from build123d import *

# Parameters (mm, degrees)
MODEL_R                 = 8.05
MODEL_W                 = 5
MODEL_H                 = 5
SALIENTE_EXTRUIR1_DEPTH = 3
CROQUIS3_W              = 20
CROQUIS3_H              = 3
SALIENTE_EXTRUIR2_DEPTH = 8
CROQUIS4_R              = 1.5
CORTAR_EXTRUIR1_DEPTH   = 3
CROQUIS5_R              = 2.25
CORTAR_EXTRUIR2_DEPTH   = 1
REDONDEO1_R             = 2
CROQUIS6_R              = 12
CORTAR_EXTRUIR3_DEPTH   = 1


with BuildPart() as part:
    # Model → Saliente-Extruir1 (new body)
    with BuildSketch(Plane.XY):
        with BuildLine():
            Line((50.698959582, -56.020997464), (70.698959582, -56.020997464))
            Line((70.698959582, -56.020997464), (70.698959582, -55.020997464))
            ThreePointArc((70.698959582, -55.020997464), (71.28474602, -53.606783901), (72.698959582, -53.020997464))
            Line((72.698959582, -53.020997464), (88.870799912, -53.020997464))
            ThreePointArc((88.870799912, -53.020997464), (90.285013474, -52.435211026), (90.870799912, -51.020997464))
            Line((90.870799912, -51.020997464), (90.870799912, 1.979002536))
            ThreePointArc((90.870799912, 1.979002536), (90.150187884, 3.212884764), (88.940527152, 3.973455574))
            ThreePointArc((88.940527152, 3.973455574), (82.556801864, 7.967186508), (80.592387516, 15.236499516))
            ThreePointArc((80.592387516, 15.236499516), (73.016137183, 12.831206377), (66.424253692, 8.389126209))
            ThreePointArc((66.424253692, 8.389126209), (62.464845981, 11.66270114), (60.387431279, 16.361376528))
            ThreePointArc((60.387431279, 16.361376528), (55.039384462, 14.426569266), (50.461877073, 11.051438157))
            ThreePointArc((50.461877073, 11.051438157), (49.41482724, 13.546636971), (50.438823204, 16.051385009))
            ThreePointArc((50.438823204, 16.051385009), (43.800023098, 13.634815248), (38.471226177, 8.99613013))
            ThreePointArc((38.471226177, 8.99613013), (37.976525569, 11.673196605), (38.618250464, 14.318872844))
            ThreePointArc((38.618250464, 14.318872844), (33.077419178, 10.94136051), (30.527119253, 4.974420659))
            Line((30.527119253, 4.974420659), (30.527119253, -51.020997464))
            ThreePointArc((30.527119253, -51.020997464), (31.112905691, -52.435211026), (32.527119253, -53.020997464))
            Line((32.527119253, -53.020997464), (48.698959582, -53.020997464))
            ThreePointArc((48.698959582, -53.020997464), (50.113173145, -53.606783901), (50.698959582, -55.020997464))
            Line((50.698959582, -55.020997464), (50.698959582, -56.020997464))
        make_face()
        with Locations((47.698959583, -8.020997464)):
            Circle(MODEL_R, mode=Mode.SUBTRACT)
        with Locations((73.698959582, -8.020997464)):
            Circle(MODEL_R, mode=Mode.SUBTRACT)
        Polygon((53.283896073, -43.364264203), (57.614023092, -45.864264203), (60.114023092, -41.534137185), (55.783896073, -39.034137185), align=None, mode=Mode.SUBTRACT)
        Polygon((63.783896073, -45.864264204), (68.114023092, -43.364264204), (65.614023092, -39.034137185), (61.283896073, -41.534137185), align=None, mode=Mode.SUBTRACT)
        with Locations((68.698959582, -35.520997464)):
            Rectangle(MODEL_W, MODEL_H, mode=Mode.SUBTRACT)
        Polygon((68.114023092, -27.677730724), (63.783896073, -25.177730724), (61.283896073, -29.507857743), (65.614023092, -32.007857743), align=None, mode=Mode.SUBTRACT)
        Polygon((57.614023092, -25.177730724), (53.283896073, -27.677730724), (55.783896073, -32.007857743), (60.114023092, -29.507857743), align=None, mode=Mode.SUBTRACT)
        with Locations((52.698959582, -35.520997464)):
            Rectangle(MODEL_W, MODEL_H, mode=Mode.SUBTRACT)
        with Locations((60.698959582, -35.520997464)):
            Rectangle(MODEL_W, MODEL_H, mode=Mode.SUBTRACT)
    extrude(amount=SALIENTE_EXTRUIR1_DEPTH)

    # Croquis3 → Saliente-Extruir2 (add)
    with BuildSketch(Plane(origin=(0, 0, 0), x_dir=(-1, 0, 0), z_dir=(0, 0, -1))):
        with Locations((-60.698959582, -54.520997464)):
            Rectangle(CROQUIS3_W, CROQUIS3_H)
    extrude(amount=SALIENTE_EXTRUIR2_DEPTH)

    # Croquis4 → Cortar-Extruir1 (cut)
    with BuildSketch(Plane(origin=(0, -53.020997464, 0), x_dir=(1, 0, 0), z_dir=(0, 1, 0))):
        with Locations((66.698959582, 3.5)):
            Circle(CROQUIS4_R)
        with Locations((54.698959582, 3.5)):
            Circle(CROQUIS4_R)
    extrude(amount=-CORTAR_EXTRUIR1_DEPTH, mode=Mode.SUBTRACT)

    # Croquis5 → Cortar-Extruir2 (cut)
    with BuildSketch(Plane(origin=(0, -53.020997464, 0), x_dir=(1, 0, 0), z_dir=(0, 1, 0))):
        with Locations((66.698959582, 3.5)):
            Circle(CROQUIS5_R)
        with Locations((54.698959582, 3.5)):
            Circle(CROQUIS5_R)
    extrude(amount=-CORTAR_EXTRUIR2_DEPTH, mode=Mode.SUBTRACT)

    # Redondeo1
    redondeo1_edges = [part.edges().sort_by_distance(p)[0] for p in [
        (50.698959582, -54.520997464, -8),
        (70.698959582, -54.520997464, -8),
    ]]
    fillet(redondeo1_edges, radius=REDONDEO1_R)

    # Croquis6 → Cortar-Extruir3 (cut)
    with BuildSketch(Plane(origin=(0, 0, 0), x_dir=(-1, 0, 0), z_dir=(0, 0, -1))):
        with Locations((-60.698959582, -35.520997464)):
            Circle(CROQUIS6_R)
    extrude(amount=-CORTAR_EXTRUIR3_DEPTH, mode=Mode.SUBTRACT)


solid = part.part
Input: part model. Units: mm. Frame: model coordinates. A direction names the side the tool comes from. Coordinates: 2 decimals unless noted, no trailing zeros. Order: outer loops, then holes, each group sorted by start corner. A loop starts at its lowest first (then second) coordinate and runs counter-clockwise, first axis right, second up. Notation, with made-up numbers: M -11,-19.5 L -7,-19.5 A15 ccw -7,-0.5 Z; hole C 47.25,75.5 d1. An arc over 180 degrees is marked long. Answer in a Markdown table with one row per item.
(1) Access query for faces 1 (the flat face through (60.9, -32.7, 1)), 2 (the flat face through (54, -54.021, -2)), 3 (the flat face through (57.919, -30.775, 1.986)), 4 (the flat face through (81, -53.021, 1)), 5 (the cylindrical face through (73.12, 12.88, 1.48)). Directions: +Z, -Z, +X, -X, +Y, -Y. A direction counts if a zero-diameter tool reaches every point of the face in a straight line with its end or side. Return the directions, or none.
Numbers:
| item | result |
|---|---|
| face 1 | -Z |
| face 2 | +Y |
| face 3 | +Z, -Z |
| face 4 | +Z, -Z, +X, -Y |
| face 5 | +Z, -Z, +Y |
(2) Section query A-A, the plane z = -3.5. Output: boundary loops of the cut face in (x, y), plus the area to 3 significant figures.
Numbers:
| item | result |
|---|---|
| outline | M 50.7,-56.02 L 53.2,-56.02 L 53.2,-54.02 L 52.45,-54.02 L 52.45,-53.02 L 50.7,-53.02 Z; M 56.2,-56.02 L 65.2,-56.02 L 65.2,-54.02 L 64.45,-54.02 L 64.45,-53.02 L 56.95,-53.02 L 56.95,-54.02 L 56.2,-54.02 Z; M 68.2,-56.02 L 70.7,-56.02 L 70.7,-53.02 L 68.95,-53.02 L 68.95,-54.02 L 68.2,-54.02 Z |
| area | 39.0 mm^2 |
(3) Section query B-B, the plane x = 79. Output: boundary loops of the cut face in (y, z), plus the area to 3 significant figures.
Numbers:
| item | result |
|---|---|
| outline | M -53.02,0 L -14.08,0 L -14.08,3 L -53.02,3 Z; M -1.96,0 L 14.92,0 L 14.92,3 L -1.96,3 Z |
| area | 167 mm^2 |
(4) Contact query for flat-ended pins moving along their axis: pin 1 Ø14.5 at (x, y) = (73.7, -8.02) entering from +Z; pin 2 Ø4 at (x, y) = (83, -37.5) entering from -Z; pin 3 Ø0.9 at (y, z) = (-54, 0.5) entering from -X; pin 4 Ø2 at (x, y) = (51.5, -30) entering from -Z. Output: stop coordinate, or through.
Numbers:
| item | result |
|---|---|
| pin 1 | passes through |
| pin 2 | stops at z = 0 |
| pin 3 | stops at x = 50.05 |
| pin 4 | stops at z = 1 |
(5) Section query C-C, the plane y = -14. Output: boundary loops of the cut face in (x, z), plus the area to 3 significant figures.
Numbers:
| item | result |
|---|---|
| outline | M 30.53,0 L 42.31,0 L 42.31,3 L 30.53,3 Z; M 53.09,0 L 68.31,0 L 68.31,3 L 53.09,3 Z; M 79.09,0 L 90.87,0 L 90.87,3 L 79.09,3 Z |
| area | 116 mm^2 |
(6) Material intervals for line 1 (X direction, y = -53.7, z = -3.5); line 2 (Y direction, x = 66.5, z = 1.5); line 3 (X direction, y = -44.5, z = 2), sorted ascending. Write a range as [from, to].
Numbers:
| item | result |
|---|---|
| line 1 | x = [50.7, 52.45], [56.95, 64.45], [68.95, 70.7] |
| line 2 | y = [-56.02, -44.3], [-40.57, -38.02], [-33.02, -30.47], [-26.75, -11.62], [-4.42, 8.46] |
| line 3 | x = [30.53, 55.25], [58.4, 63], [66.15, 90.87] |
(7) Section query D-D, the plane y = -1.5. Output: boundary loops of the cut face in (x, z).
Numbers:
| item | result |
|---|---|
| outline | M 30.53,0 L 42.98,0 L 42.98,3 L 30.53,3 Z; M 52.42,0 L 68.98,0 L 68.98,3 L 52.42,3 Z; M 78.42,0 L 90.87,0 L 90.87,3 L 78.42,3 Z |
(8) Draft query along Y for faces 6 (the cylindrical face through (65.2, -55.01, -3.57)), 7 (the flat face through (61, -56.021, -2)), 8 (the flat face through (66.85, -29.87, 1.99)). Return one class per face: pulls with the +Y half, pulls with the -Y half, needs draft (parallel to the pull), parting line crosses it, or undercut.
Numbers:
| item | result |
|---|---|
| face 6 | needs draft |
| face 7 | pulls with the -Y half |
| face 8 | undercut |
